The model under review builds one solid part; all positions refer to its coordinate system, in mm. Face numbers are marked on the shaded views. A direction names the side the tool comes from. Round coordinates to 2 decimals unless told otherwise and drop trailing zeros. Write each loop counter-clockwise with the first axis right and the second up, starting at its lowest first coordinate (ties: lowest second). Pieces come first, ordered by that corner, then holes. Notation, with made-up numbers: M -14.75,40.25 L 1.25,40.25 A36 cw 1.25,76.25 Z; hole C -15,73.25 d3. An arc over 180 degrees is marked long. Write item = value, one per line. Start each with the question number.
Item 1: Take a section at C-C, the plane z = 10. Give the boundary of the cut face in (x, y), plus the area to 3 significant figures.
Item 2: Take a section at D-D, the plane y = -3.25. Give the boundary of the cut face in (x, z).
Item 3: To check wall thickness, follow line 1 along Z through (x, y) = (0, -6.5); line 2 along Y through (x, z) = (-7, -20.5); line 3 along Z through (x, y) = (-41, -6.75). State the ranges of each line that lie inside material, in increasing order.
Item 4: Tool access review of the marked faces 1, 2 and 3: name each direction out of +Z, -Z, +X, -X, +Y, -Y from which nothing blocks a thin tool from reaching the whole face with its end or side.
Item 5: The part is to be moulded in two halves that separate along X. For the marked faces 4, 5, 6 and 7, say which applies: +X half, -X half, draft (parallel to the pull), parting line (faces both ways), or undercut.
Item 6: Take a section at A-A, the plane y = -9. Give the boundary of the cut face in (x, z), plus the area to 3 significant figures.
Item 7: For pin 1 Ø16 at (x, z) = (0, -12.7) entering from +Y; pin 2 Ø12.5 at (x, y) = (-15, 3.5) entering from +Z; pin 3 Ø6 at (y, z) = (2.5, -20.5) entering from +X; pin 4 Ø1 at (x, z) = (-12.5, 7.5) entering from +Y, all flat-tipped, find the tip position at first contact; note any pin that passes through.
Item 8: Take a section at B-B, the plane x = -0.5. Give the boundary of the cut face in (y, z).
from build123d import *

# Parameters (mm, degrees)
F0_R     = 4.953
F1_DEPTH = 12.7
F2_W     = 64.77
F2_H     = 9.906
F3_DEPTH = 24.639


with BuildPart() as f1:
    # F0 (on Front) → F1 (new body, symmetric)
    with BuildSketch(Plane.XZ):
        with BuildLine():
            Line((-39.624, 12.7), (-52.07, 12.7))
            Line((-52.07, 12.7), (-52.07, 0))
            Line((-52.07, 0), (-5.699577, -23.287221))
            ThreePointArc((-5.699577, -23.287221), (6.667285, -22.747131), (12.7, -11.938))
            Line((12.7, -11.938), (12.7, 0))
            Line((12.7, 0), (12.7, 12.7))
            Line((12.7, 12.7), (0.254, 12.7))
            Line((0.254, 12.7), (6.096, 6.858))
            Line((6.096, 6.858), (-45.466, 6.858))
            Line((-45.466, 6.858), (-39.624, 12.7))
        make_face()
        with Locations((0, -12.7)):
            Circle(F0_R, mode=Mode.SUBTRACT)
    extrude(amount=F1_DEPTH, both=True)

    # F2 (on Top) → F3 (cut, through all)
    with BuildSketch(Plane.XY):
        with Locations((-19.685, 0)):
            Rectangle(F2_W, F2_H)
    extrude(amount=-F3_DEPTH, mode=Mode.SUBTRACT)


solid = f1.part
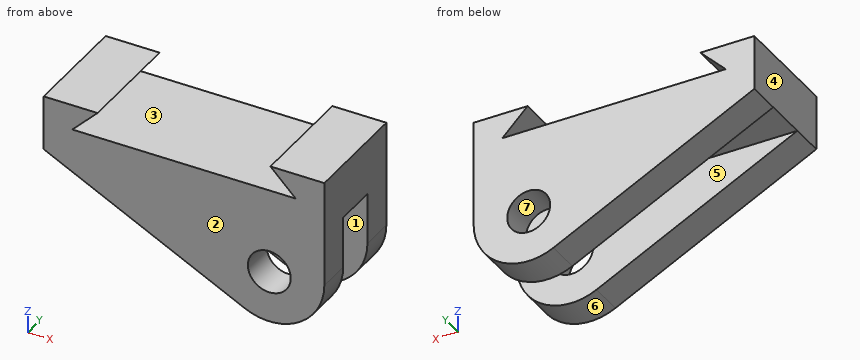
Response values:
q1.outline = M -52.07,-12.7 L -42.32,-12.7 L -42.32,12.7 L -52.07,12.7 Z; M 2.95,-12.7 L 12.7,-12.7 L 12.7,12.7 L 2.95,12.7 Z
q1.area = 495 mm2
q2.outline = M -52.07,0 L 12.7,0 L 12.7,12.7 L 0.25,12.7 L 6.1,6.86 L -45.47,6.86 L -39.62,12.7 L -52.07,12.7 Z
q3.line_1 = -24.64 to -17.65, -7.75 to 6.86
q3.line_2 = -12.7 to -4.95, 4.95 to 12.7
q3.line_3 = -5.56 to 6.86, 11.32 to 12.7
q4.face_1 = -Z, +X, -X
q4.face_2 = +Z, -Z, +X, -X, -Y
q4.face_3 = +Y, -Y
q5.face_4 = -X half
q5.face_5 = draft
q5.face_6 = parting line
q5.face_7 = undercut
q6.outline = M -52.07,0 L -5.7,-23.29 A12.7 ccw 12.7,-11.94 L 12.7,12.7 L 0.25,12.7 L 6.1,6.86 L -45.47,6.86 L -39.62,12.7 L -52.07,12.7 Z; hole C 0,-12.7 d9.91
q6.area = 1,430 mm2
q7.pin_1 = 12.7
q7.pin_2 = 6.86
q7.pin_3 = 10.7
q7.pin_4 = through
q8.outline = M -12.7,-24.63 L -4.95,-24.63 L -4.95,-17.63 L -12.7,-17.63 Z; M -12.7,-7.77 L -4.95,-7.77 L -4.95,0 L 4.95,0 L 4.95,-7.77 L 12.7,-7.77 L 12.7,6.86 L -12.7,6.86 Z; M 4.95,-24.63 L 12.7,-24.63 L 12.7,-17.63 L 4.95,-17.63 Z
